from build123d import *

# Parameters (mm, degrees)
SKETCH1_W           = 700
SKETCH1_H           = 50
SKETCH1_W_2         = 50
SKETCH1_R           = 5
SKETCH1_H_2         = 160
BOSS_EXTRUDE1_DEPTH = 3
FILLET1_R           = 20
EDGE_FLANGE1_DEPTH  = 760
CUT_EXTRUDE1_START  = 80
CUT_EXTRUDE1_DEPTH  = 650


# Read off the part's stored shape, not the designer's step: Cut-Extrude1
# Sheet-metal steps are written as plain solids
with BuildPart() as part:
    # Sketch1 → Boss-Extrude1 (new body)
    # profile 1 of 5: a face of its own
    with BuildSketch(Plane.XY):
        with Locations((350, 25)):
            Rectangle(SKETCH1_W, SKETCH1_H)
    # profile 2 of 5: a face of its own
    with BuildSketch(Plane.XY):
        with Locations((-25, 25)):
            Rectangle(SKETCH1_W_2, SKETCH1_H)
    # profile 3 of 5: a face of its own
    with BuildSketch(Plane.XY):
        Polygon((-50, -55), (-50, 0), (-50, 50), (-50, 105), (-100, 105), (-100, -55), align=None)
        with Locations((-75, -35)):
            Circle(SKETCH1_R, mode=Mode.SUBTRACT)
        with Locations((-75, 85)):
            Circle(SKETCH1_R, mode=Mode.SUBTRACT)
    # profile 4 of 5: a face of its own
    with BuildSketch(Plane.XY):
        with Locations((775, 25)):
            Rectangle(SKETCH1_W_2, SKETCH1_H_2)
        with Locations((775, -35)):
            Circle(SKETCH1_R, mode=Mode.SUBTRACT)
        with Locations((775, 85)):
            Circle(SKETCH1_R, mode=Mode.SUBTRACT)
    # profile 5 of 5: a face of its own
    with BuildSketch(Plane.XY):
        with Locations((725, 25)):
            Rectangle(SKETCH1_W_2, SKETCH1_H)
    extrude(amount=BOSS_EXTRUDE1_DEPTH)

    # Fillet1
    fillet1_edges = [part.edges().sort_by_distance(p)[0] for p in [
        (-50, 0, 1.5),
        (-50, -55, 1.5),
        (-100, -55, 1.5),
        (-100, 105, 1.5),
        (-50, 105, 1.5),
        (-50, 50, 1.5),
        (750, 50, 1.5),
        (750, 105, 1.5),
        (800, 105, 1.5),
        (800, -55, 1.5),
        (750, -55, 1.5),
        (750, 0, 1.5),
    ]]
    fillet(fillet1_edges, radius=FILLET1_R)

    # Edge-Flange1 section (across the edge) → Edge-Flange1 (add)
    with BuildSketch(Plane(origin=(-30, -2, 3), x_dir=(0, 1, 0), z_dir=(1, 0, 0))):
        with BuildLine():
            Line((-3, 2), (-3, 67))
            Line((-3, 67), (0, 67))
            Line((0, 67), (0, 2))
            ThreePointArc((0, 2), (0.585786438, 0.585786438), (2, 0))
            Line((2, 0), (2, -3))
            ThreePointArc((2, -3), (-1.535533906, -1.535533906), (-3, 2))
        make_face()
    extrude(amount=EDGE_FLANGE1_DEPTH)

    # Cut-Extrude1 outline → Cut-Extrude1 (cut)
    with BuildSketch(Plane.YZ.offset(CUT_EXTRUDE1_START)):
        with BuildLine():
            ThreePointArc((-5, 5), (-4.183300133, 2.261387212), (-2, 0.417424305))
            Line((-2, 0.417424305), (-0.8, 3.166969722))
            ThreePointArc((-0.8, 3.166969722), (-1.673320053, 3.904554885), (-2, 5))
            Line((-2, 5), (-2, 70))
            Line((-2, 70), (-5, 70))
            Line((-5, 70), (-5, 5))
        make_face()
    extrude(amount=CUT_EXTRUDE1_DEPTH, mode=Mode.SUBTRACT)


solid = part.part
Could you check a few things on this model? Use its own coordinates, in mm. A direction names the side the tool comes from. Round coordinates to 2 decimals unless told otherwise and drop trailing zeros. Write each loop counter-clockwise with the first axis right and the second up, starting at its lowest first coordinate (ties: lowest second). Pieces come first, ordered by that corner, then holes. Notation, with made-up numbers: (8.25, 12) -> (30.25, 12) arc R20 ccw to (30.25, 36) -> close; hole circle Ø8 at (74, 60.5). An arc over 180 degrees is marked (long way). Use a Markdown table: item, result.
1. If we section it at D-D (x = 256): List the corners of the cut face in (y, z) for me, then the cut area to 3 significant figures.
Answer key:
| item | result |
|---|---|
| outline | (-2, 0.42) arc R5 ccw to (0, 0) -> (50, 0) -> (50, 3) -> (0, 3) arc R2 cw to (-0.8, 3.17) -> close |
| area | 154 mm^2 |
2. We'd pull the mould along X, two halves only. Please class faces 1 (the face through (-94.297, 98.986, 1.521)), 2 (the face through (756.014, -49.297, 1.521)), 3 (the face through (244, 26, 3)): +X half, -X half, draft (parallel to the pull), parting line (faces both ways), or undercut.
Answer key:
| item | result |
|---|---|
| face 1 | -X half |
| face 2 | undercut |
| face 3 | draft |
3. For pin 1 Ø1.3 at (y, z) = (-2, 37) entering from +X; pin 2 Ø19.5 at (x, z) = (30.5, 30.5) entering from +Y; pin 3 Ø5 at (y, z) = (-1.5, 32.5) entering from -X; pin 4 Ø9 at (x, y) = (775, 85) entering from -Z, each with a flat end and sliding along its axis, tell me the tip position at first contact or that it passes through.
Answer key:
| item | result |
|---|---|
| pin 1 | stops at x = 80 |
| pin 2 | stops at y = -2 |
| pin 3 | stops at x = -30 |
| pin 4 | passes through |
4. Which directions (+Z, -Z, +X, -X, +Y, -Y) give clear straight access to the entire face, cutting with the end or side of a thin tool? Please do faces 4 (the face through (24, -2, 38)), 5 (the face through (244, 26, 0)), 6 (the face through (-56.014, 99.297, 1.521)), 7 (the face through (-56.014, -49.297, 1.521)).
Answer key:
| item | result |
|---|---|
| face 4 | +Z, +X, -X, +Y |
| face 5 | -Z, +X, -X, +Y, -Y |
| face 6 | +Z, -Z, +Y |
| face 7 | +Z, -Z, -Y |
5. Please list where these lines run through material, in increasing order: probe 1 along Y at (x, z) = (775, 1.95); probe 2 along Z at (x, y) = (353, 6); probe 3 along Z at (x, y) = (20, -3).
Answer key:
| item | result |
|---|---|
| probe 1 | y = -55 to -40, -30 to 80, 90 to 105 |
| probe 2 | z = 0 to 3 |
| probe 3 | z = 1 to 70 |
6. If we section it at C-C (y = 37): List the corners of the cut face in (x, z) for me, then the cut area to 3 significant figures.
Answer key:
| item | result |
|---|---|
| outline | (-100, 0) -> (800, 0) -> (800, 3) -> (-100, 3) -> close |
| area | 2,700 mm^2 |
7. If we section it at B-B (z = 22): List the corners of the cut face in (x, y) for me, then the cut area to 3 significant figures.
Answer key:
| item | result |
|---|---|
| outline | (-30, -5) -> (80, -5) -> (80, -2) -> (-30, -2) -> close |
| area | 330 mm^2 |
8. If we section it at A-A (x = 49): List the corners of the cut face in (y, z) for me.
Answer key:
| item | result |
|---|---|
| outline | (-5, 5) arc R5 ccw to (0, 0) -> (50, 0) -> (50, 3) -> (0, 3) arc R2 cw to (-2, 5) -> (-2, 70) -> (-5, 70) -> close |
